Verification items for this drawing (mm, ordinates from the low corner). Give positions to 0.01 mm unless a question says otherwise; leave off trailing zeros. Order: outer loops, then holes, each group sorted by start corner. A loop starts at its lowest first (then second) coordinate and runs counter-clockwise, first axis right, second up.
(1) Mould release check, pull along Y, two halves, no side actions. Record for the marked faces 1, 2 and 3: pulls with the +Y half, pulls with the -Y half, needs draft (parallel to the pull), parting line crosses it, or undercut.
(2) Gauge pin test, flat ends, axial feed: pin 1 (1 mm diameter, centred on x = 2, z = 1, fed in from -Y); pin 2 (2 mm diameter, centred on x = 4.5, z = 2, fed in from -Y). Record the tip position at first contact, or that the pin passes through.
(3) Sectioned sample at D-D on z = 0.3. Record the cut outline in (x, y).
(4) Sectioned sample at C-C on z = 4.65. Record the cut outline in (x, y).
(5) Scan lines: L1, parallel to X at y = 2.5, z = 2.4; L2, parallel to X at y = 2.5, z = 1.6. Record each from-to range of solid material in increasing order.
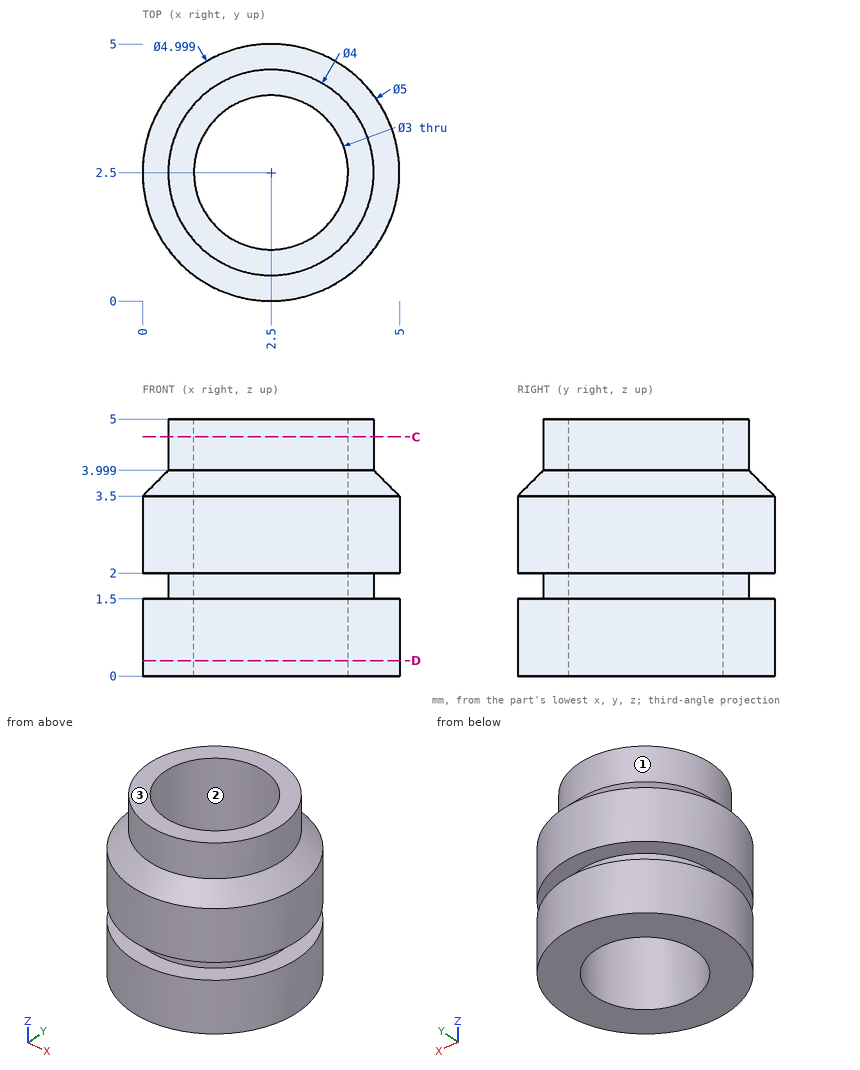
Ans:
1. face 1: parting line crosses it
1. face 2: undercut
1. face 3: needs draft
2. pin 1: stops at y = 0
2. pin 2: stops at y = 0.21
3. outline: circle Ø5 at (2.5, 2.5); hole circle Ø3 at (2.5, 2.5)
4. outline: circle Ø4 at (2.5, 2.5); hole circle Ø3 at (2.5, 2.5)
5. L1: x = 0 to 1, 4 to 5
5. L2: x = 0.5 to 1, 4 to 4.5
